```python
from build123d import *

# Parameters (mm, degrees)
F0_W     = 3.175
F0_H     = 48.4495080546
F0_W_2   = 3.4043772995
F1_DEPTH = 6.35


# Not quite as in the source:
# - a feature names something its author has since deleted; it is built from what else it names


with BuildPart() as f1:
    # F0 (on Front) → F1 (new body)
    with BuildSketch(Plane.XZ):
        Polygon((12.7, -44.45), (57.1500004709, -44.45), (63.5, -44.45), (63.5, -12.7), (57.1500004709, -12.7), (57.1500004709, -1.4605), (52.7050002354, -1.4605), (52.7050002354, -2.69367), (50.1650002354, -2.69367), (50.1650002354, -1.4605), (45.72, -1.4605), (45.72, 1.4605), (50.1650002354, 1.4605), (50.1650002354, 2.69367), (52.7050002354, 2.69367), (52.7050002354, 1.4605), (57.1500004709, 1.4605), (57.1500004709, 12.7), (63.5, 12.7), (63.5, 44.45), (57.1500004709, 44.45), (12.7, 44.45), (12.7, 38.1000004709), (1.4605, 38.1000004709), (1.4605, 33.6550002354), (2.69367, 33.6550002354), (2.69367, 31.1150002354), (1.4605, 31.1150002354), (1.4605, 26.67), (-1.4605, 26.67), (-1.4605, 31.1150002354), (-2.69367, 31.1150002354), (-2.69367, 33.6550002354), (-1.4605, 33.6550002354), (-1.4605, 38.1000004709), (-12.7, 38.1000004709), (-12.7, 44.45), (-57.1500004709, 44.45), (-63.5, 44.45), (-63.5, 12.7), (-57.1500004709, 12.7), (-57.1500004709, 1.4605), (-52.7050002354, 1.4605), (-52.7050002354, 2.69367), (-50.1650002354, 2.69367), (-50.1650002354, 1.4605), (-45.72, 1.4605), (-45.72, -1.4605), (-50.1650002354, -1.4605), (-50.1650002354, -2.69367), (-52.7050002354, -2.69367), (-52.7050002354, -1.4605), (-57.1500004709, -1.4605), (-57.1500004709, -2.69367), (-57.1500004709, -12.7), (-63.5, -12.7), (-63.5, -44.45), (-57.1500004709, -44.45), (-12.7, -44.45), (-12.7, -38.1000004709), (-1.4605, -38.1000004709), (-1.4605, -33.6550002354), (-2.69367, -33.6550002354), (-2.69367, -31.1150002354), (-1.4605, -31.1150002354), (-1.4605, -26.67), (1.4605, -26.67), (1.4605, -31.1150002354), (2.69367, -31.1150002354), (2.69367, -33.6550002354), (1.4605, -33.6550002354), (1.4605, -38.1000004709), (12.7, -38.1000004709), align=None)
        with Locations((-33.3375002354, 4.3502459727)):
            Rectangle(F0_W, F0_H, mode=Mode.SUBTRACT)
        with Locations((-26.9875002354, 4.3502459727)):
            Rectangle(F0_W, F0_H, mode=Mode.SUBTRACT)
        with Locations((-20.5228115857, 4.3502459727)):
            Rectangle(F0_W_2, F0_H, mode=Mode.SUBTRACT)
        with Locations((-14.1728115857, 4.3502459727)):
            Rectangle(F0_W_2, F0_H, mode=Mode.SUBTRACT)
        Polygon((0.2293770641, -19.8745080546), (-3.1750002354, -19.8745080546), (-3.1750002354, 24.4311112911), (0, 24.4311112911), align=None, mode=Mode.SUBTRACT)
        with Locations((-7.8228115857, 4.3502459727)):
            Rectangle(F0_W_2, F0_H, mode=Mode.SUBTRACT)
        with Locations((4.8771884143, 4.3502459727)):
            Rectangle(F0_W_2, F0_H, mode=Mode.SUBTRACT)
        with Locations((11.2271884143, 4.3502459727)):
            Rectangle(F0_W_2, F0_H, mode=Mode.SUBTRACT)
        with Locations((17.5771884143, 4.3502459727)):
            Rectangle(F0_W_2, F0_H, mode=Mode.SUBTRACT)
        with Locations((23.9271884143, 4.3502459727)):
            Rectangle(F0_W_2, F0_H, mode=Mode.SUBTRACT)
        with Locations((30.2771884143, 4.3502459727)):
            Rectangle(F0_W_2, F0_H, mode=Mode.SUBTRACT)
    extrude(amount=F1_DEPTH)


solid = f1.part
```
Source: CAD feature listing. Evaluate the final solid. Frame: model axes, mm. A direction names the side the tool comes from. Give positions to 0.01 mm unless a question says otherwise; leave off trailing zeros. Order: outer loops, then holes, each group sorted by start corner. A loop starts at its lowest first (then second) coordinate and runs counter-clockwise, first axis right, second up.
(1) Access query for faces 4 (the face through (31.979, -3, 4)), 5 (the face through (60, -3, 12.7)), 6 (the face through (-48, -3, -1.46)), 7 (the face through (1.46, -3, 29)). Directions: +Z, -Z, +X, -X, +Y, -Y. A direction counts if a zero-diameter tool reaches every point of the face in a straight line with its end or side. Return the directions, or none.
(2) Pull-direction query (Z, two-part tool) for faces 1 (the face through (1.46, -3, -36)), 2 (the face through (-38, -3, -44.45)), 3 (the face through (11, -3, -19.875)); classes: +Z half, -Z half, draft (parallel to the pull), parting line (faces both ways), or undercut.
(3) Section query B-B (z = 36.5). Return the cut outline in (x, y).
(4) Section query A-A (x = -54.5). Return the cut outline in (y, z).
(5) Contact query for flat-ended pins moving along their axis: P1, Ø1.9, axis at x = -6.5, y = -4.5, coming from the -Z side; P2, Ø1.4, axis at x = -2, y = -4.5, coming from the +Z side; P3, Ø0.6, axis at y = -2.5, z = -2, coming from the +X side. Output: stop coordinate, or through.
(6) Section query C-C (y = -4.75). State how many separate pieces and enclosed holes the cut face has, plus the area to 3 significant figures.
(7) Material intervals for line 1 along Z through (x, y) = (54, -1); line 2 along X through (y, z) = (-2.75, 35.5); line 3 along Z through (x, y) = (10, -0.75) (1 decimal), sorted ascending.
Outcome:
1. face 4: +Y, -Y
1. face 5: +X, +Y, -Y
1. face 6: -X, +Y, -Y
1. face 7: +Z, +Y, -Y
2. face 1: draft
2. face 2: -Z half
2. face 3: undercut
3. outline: (-63.5, -6.35) - (-1.46, -6.35) - (-1.46, 0) - (-63.5, 0) - close; (1.46, -6.35) - (63.5, -6.35) - (63.5, 0) - (1.46, 0) - close
4. outline: (-6.35, -44.45) - (0, -44.45) - (0, -1.46) - (-6.35, -1.46) - close; (-6.35, 1.46) - (0, 1.46) - (0, 44.45) - (-6.35, 44.45) - close
5. P1: stops at z = -38.1
5. P2: stops at z = 38.1
5. P3: stops at x = 57.15
6. separate pieces: 1
6. enclosed holes: 11
6. area: 8,710 mm2
7. line 1: z = -44.45 to -1.46, 1.46 to 44.45
7. line 2: x = -63.5 to -1.46, 1.46 to 63.5
7. line 3: z = -38.1 to -19.9, 28.6 to 38.1
